```python
from build123d import *

# Parameters (mm, degrees)
SKETCH1_W                      = 96
SKETCH1_H                      = 96
BOSS_EXTRUDE1_DEPTH            = 8
SKETCH2_W                      = 92
SKETCH2_H                      = 92
COMPONENT_PLATFORM_DEPTH       = 6
CABLE_SLOTS_DEPTH              = 6
SKETCH4_R                      = 7.5
CENTER_MASS_CUT_DEPTH          = 6
INNER_CORNER_FILLETS_R         = 3
SKETCH10_W                     = 11
SKETCH10_H                     = 10
MOTOR_CUTOUT_DEPTH             = 2
FILLET1_R                      = 3
M3X0_5_TAPPED_HOLE1_AT_2_COUNT = 2
M3X0_5_TAPPED_HOLE1_AT_2_PITCH = 70
M3X0_5_TAPPED_HOLE2_AT_2_COUNT = 2
M3X0_5_TAPPED_HOLE2_AT_2_PITCH = 70
M2X0_4_TAPPED_HOLE1_D          = 1.6
M2X0_4_TAPPED_HOLE1_DEPTH      = 5.2
M2X0_4_TAPPED_HOLE1_TIP        = 0.480688495


with BuildPart() as part:
    # Sketch1 → Boss-Extrude1 (new body)
    with BuildSketch(Plane.XY):
        Rectangle(SKETCH1_W, SKETCH1_H)
    extrude(amount=BOSS_EXTRUDE1_DEPTH)

    # Sketch2 → Component Platform (cut)
    with BuildSketch(Plane.XY.offset(8)):
        Rectangle(SKETCH2_W, SKETCH2_H)
    extrude(amount=-COMPONENT_PLATFORM_DEPTH, mode=Mode.SUBTRACT)

    # Sketch3 → Cable Slots (cut, symmetric)
    with BuildSketch(Plane.XY.offset(2)):
        with BuildLine():
            Line((-33.878679656, -25.121320344), (-28.878679656, -20.121320344))
            ThreePointArc((-28.878679656, -20.121320344), (-28.228361402, -19.148050297), (-28, -18))
            Line((-28, -18), (-28, 18))
            ThreePointArc((-28, 18), (-28.228361402, 19.148050297), (-28.878679656, 20.121320344))
            Line((-28.878679656, 20.121320344), (-33.878679656, 25.121320344))
            ThreePointArc((-33.878679656, 25.121320344), (-34.851949703, 25.771638598), (-36, 26))
            Line((-36, 26), (-48, 26))
            Line((-48, 26), (-48, -26))
            Line((-48, -26), (-36, -26))
            ThreePointArc((-36, -26), (-34.851949703, -25.771638598), (-33.878679656, -25.121320344))
        make_face()
        with BuildLine():
            Line((48, -26), (48, 26))
            Line((48, 26), (36, 26))
            ThreePointArc((36, 26), (34.851949703, 25.771638598), (33.878679656, 25.121320344))
            Line((33.878679656, 25.121320344), (28.878679656, 20.121320344))
            ThreePointArc((28.878679656, 20.121320344), (28.228361402, 19.148050297), (28, 18))
            Line((28, 18), (28, -18))
            ThreePointArc((28, -18), (28.228361402, -19.148050297), (28.878679656, -20.121320344))
            Line((28.878679656, -20.121320344), (33.878679656, -25.121320344))
            ThreePointArc((33.878679656, -25.121320344), (34.851949703, -25.771638598), (36, -26))
            Line((36, -26), (48, -26))
        make_face()
    extrude(amount=CABLE_SLOTS_DEPTH, both=True, mode=Mode.SUBTRACT)

    # Sketch4 → Center Mass Cut (cut)
    with BuildSketch(Plane.XY.offset(2)):
        Circle(SKETCH4_R)
    extrude(amount=-CENTER_MASS_CUT_DEPTH, mode=Mode.SUBTRACT)

    # Inner Corner Fillets
    inner_corner_fillets_edges = [part.edges().sort_by_distance(p)[0] for p in [
        (-46, -46, 5),
        (-46, 46, 5),
        (46, 46, 5),
        (46, -46, 5),
    ]]
    fillet(inner_corner_fillets_edges, radius=INNER_CORNER_FILLETS_R)

    # Sketch10 → Motor Cutout (cut)
    with BuildSketch(Plane.XY.offset(2)):
        with Locations((5.5, 0)):
            Rectangle(SKETCH10_W, SKETCH10_H)
    extrude(amount=-MOTOR_CUTOUT_DEPTH, mode=Mode.SUBTRACT)

    # Fillet1
    fillet1_edges = [part.edges().sort_by_distance(p)[0] for p in [
        (11, -5, 1),
        (11, 5, 1),
    ]]
    fillet(fillet1_edges, radius=FILLET1_R)

    # Sketch14 → M3x0.5 Tapped Hole1 (revolve, cut)
    with BuildSketch(Plane(origin=(48, -35, 5), x_dir=(0, 0, -1), z_dir=(0, 1, 0))):
        Polygon((0, 0), (0, 8.251075774), (1.25, 7.5), (1.25, 0), align=None)
    m3x0_5_tapped_hole1 = revolve(axis=Axis((54.35, -35, 5), (-1, 0, 0)), mode=Mode.SUBTRACT)

    # M3x0.5 Tapped Hole1 at 2: M3x0.5 Tapped Hole1 ×2
    with Locations(*[(0, i * M3X0_5_TAPPED_HOLE1_AT_2_PITCH, 0) for i in range(1, M3X0_5_TAPPED_HOLE1_AT_2_COUNT)]):
        add(m3x0_5_tapped_hole1, mode=Mode.SUBTRACT)

    # Sketch17 → M3x0.5 Tapped Hole2 (revolve, cut)
    with BuildSketch(Plane(origin=(35, 48, 5), x_dir=(0, 0, 1), z_dir=(1, 0, 0))):
        Polygon((0, 0), (0, 8.251075774), (1.25, 7.5), (1.25, 0), align=None)
    m3x0_5_tapped_hole2 = revolve(axis=Axis((35, 54.35, 5), (0, -1, 0)), mode=Mode.SUBTRACT)

    # M3x0.5 Tapped Hole2 at 2: M3x0.5 Tapped Hole2 ×2
    with Locations(*[(-i * M3X0_5_TAPPED_HOLE2_AT_2_PITCH, 0, 0) for i in range(1, M3X0_5_TAPPED_HOLE2_AT_2_COUNT)]):
        add(m3x0_5_tapped_hole2, mode=Mode.SUBTRACT)

    # Mirror1: M3x0.5 Tapped Hole1 across plane
    add(m3x0_5_tapped_hole1.mirror(Plane(origin=(0, 0, 0), x_dir=(0, 0, 1), z_dir=(1, 0, 0))), mode=Mode.SUBTRACT)

    # Mirror1 copy 1 sketch → Mirror1 copy 1 (revolve, cut)
    with BuildSketch(Plane(origin=(-48, 35, 5), x_dir=(0, 0, -1), z_dir=(0, 1, 0))):
        Polygon((0, 0), (0, -8.251075774), (1.25, -7.5), (1.25, 0), align=None)
    revolve(axis=Axis((-54.35, 35, 5), (-1, 0, 0)), mode=Mode.SUBTRACT)

    # Mirror2: M3x0.5 Tapped Hole2 across plane
    add(m3x0_5_tapped_hole2.mirror(Plane(origin=(0, 0, 0), x_dir=(0, 0, 1), z_dir=(0, -1, 0))), mode=Mode.SUBTRACT)

    # Mirror2 copy 1 sketch → Mirror2 copy 1 (revolve, cut)
    with BuildSketch(Plane(origin=(-35, -48, 5), x_dir=(0, 0, 1), z_dir=(1, 0, 0))):
        Polygon((0, 0), (0, -8.251075774), (1.25, -7.5), (1.25, 0), align=None)
    revolve(axis=Axis((-35, -54.35, 5), (0, -1, 0)), mode=Mode.SUBTRACT)

    # Sketch20 → M3x0.5 Tapped Hole3 (revolve, cut)
    with BuildSketch(Plane(origin=(-28.5, -28.5, 2), x_dir=(0, -1, 0), z_dir=(1, 0, 0))):
        Polygon((0, 0), (0, 8.251075774), (1.25, 7.5), (1.25, 0), align=None)
    m3x0_5_tapped_hole3 = revolve(axis=Axis((-28.5, -28.5, 8.35), (0, 0, -1)), mode=Mode.SUBTRACT)

    # Mirror3: M3x0.5 Tapped Hole3 across plane
    add(m3x0_5_tapped_hole3.mirror(Plane(origin=(0, 0, 0), x_dir=(0, 0, 1), z_dir=(1, 0, 0))), mode=Mode.SUBTRACT)

    # Mirror4: M3x0.5 Tapped Hole3 across plane
    add(m3x0_5_tapped_hole3.mirror(Plane.ZX), mode=Mode.SUBTRACT)

    # Mirror4 copy 1 sketch → Mirror4 copy 1 (revolve, cut)
    with BuildSketch(Plane(origin=(28.5, 28.5, 2), x_dir=(0, 1, 0), z_dir=(-1, 0, 0))):
        Polygon((0, 0), (0, 8.251075774), (1.25, 7.5), (1.25, 0), align=None)
    revolve(axis=Axis((28.5, 28.5, 8.35), (0, 0, -1)), mode=Mode.SUBTRACT)

    # M2x0.4 Tapped Hole1
    with Locations(Plane.XY.offset(2)):
        with Locations((6.72, -6.72), (0, -10), (-6.72, -6.72), (-10, 0), (-6.72, 6.72), (0, 10), (6.72, 6.72)):
            Hole(M2X0_4_TAPPED_HOLE1_D / 2, depth=M2X0_4_TAPPED_HOLE1_DEPTH)
            with Locations((0, 0, -(M2X0_4_TAPPED_HOLE1_DEPTH + M2X0_4_TAPPED_HOLE1_TIP / 2))):  # 118° drill point
                Cone(0, M2X0_4_TAPPED_HOLE1_D / 2, M2X0_4_TAPPED_HOLE1_TIP, mode=Mode.SUBTRACT)


solid = part.part
```
Verification items for the finished model (mm, model axes). A direction names the side the tool comes from. Coordinates: 2 decimals unless noted, no trailing zeros. Write each loop counter-clockwise with the first axis right and the second up, starting at its lowest first coordinate (ties: lowest second). Pieces come first, ordered by that corner, then holes. Notation, with made-up numbers: M -5,-35.5 L 21,-35.5 A18 cw 21,-26.5 Z; hole C 65.5,64 d6. An arc over 180 degrees is marked long. One line per item, written item: value.
Item 1: Section check B-B, the plane x = 4. Record the boundary of the cut face in (y, z).
Check sheet entries:
outline: M -48,0 L -6.34,0 L -6.34,2 L -46,2 L -46,8 L -48,8 Z; M 6.34,0 L 48,0 L 48,8 L 46,8 L 46,2 L 6.34,2 Z
Item 2: Section check C-C, the plane x = 17. Record the boundary of the cut face in (y, z), plus the area to 3 significant figures.
Check sheet entries:
outline: M -48,0 L 48,0 L 48,8 L 46,8 L 46,2 L -46,2 L -46,8 L -48,8 Z
area: 216 mm^2
Item 3: Section check D-D, the plane x = 32. Record the boundary of the cut face in (y, z), plus the area to 3 significant figures.
Check sheet entries:
outline: M -48,0 L -23.24,0 L -23.24,2 L -46,2 L -46,8 L -48,8 Z; M 23.24,0 L 48,0 L 48,8 L 46,8 L 46,2 L 23.24,2 Z
area: 123 mm^2
Item 4: Section check A-A, the plane y = -28.5. Record the boundary of the cut face in (x, z), plus the area to 3 significant figures.
Check sheet entries:
outline: M -48,0 L -29.75,0 L -29.75,2 L -46,2 L -46,8 L -48,8 Z; M -27.25,0 L 27.25,0 L 27.25,2 L -27.25,2 Z; M 29.75,0 L 48,0 L 48,8 L 46,8 L 46,2 L 29.75,2 Z
area: 206 mm^2
Item 5: Scan lines: line 1 along Y through (x, z) = (0, 1.35); line 2 along X through (y, z) = (-28.5, 1.55); line 3 along X through (y, z) = (47.25, 5). Record each from-to range of solid material in increasing order.
Check sheet entries:
line 1: y = -48 to -10.8, -9.2 to -7.5, 7.5 to 9.2, 10.8 to 48
line 2: x = -48 to -29.75, -27.25 to 27.25, 29.75 to 48
line 3: x = -48 to -36.25, -33.75 to 33.75, 36.25 to 48
Item 6: Gauge pin test, flat ends, axial feed: pin 1 Ø8 at (x, y) = (10.5, 13) entering from +Z; pin 2 Ø1.4 at (x, y) = (-6.72, -6.72) entering from +Z; pin 3 Ø1.5 at (y, z) = (-18, 1) entering from +X; pin 4 Ø2 at (y, z) = (2.5, 1) entering from +X. Record the tip position at first contact, or that the pin passes through.
Check sheet entries:
pin 1: stops at z = 2
pin 2: passes through
pin 3: stops at x = 28.1
pin 4: stops at x = 28
Item 7: Access from +Z, -Z, +X, -X, +Y, -Y to the whole of each face (thin tool, end or side, straight path). Record for faces 5 (the flat face through (46, 34, 4)), 6 (the cylindrical face through (10.14, 4.1, 0.99)), 7 (the flat face through (-31.414, -22.656, 0.986)).
Check sheet entries:
face 5: +Z
face 6: +Z, -Z
face 7: +Z, -Z, -X
Item 8: Mould release check, pull along X, two halves, no side actions. Record for faces 1 (the cylindrical face through (45.14, 45.1, 4.96)), 2 (the cylindrical face through (-33.78, -47.01, 4.73)), 3 (the flat face through (31.414, 22.656, 1.014)), 4 (the flat face through (-48, -37, 4)): pulls with the +X half, pulls with the -X half, needs draft (parallel to the pull), parting line crosses it, or undercut.
Check sheet entries:
face 1: undercut
face 2: undercut
face 3: pulls with the +X half
face 4: pulls with the -X half
